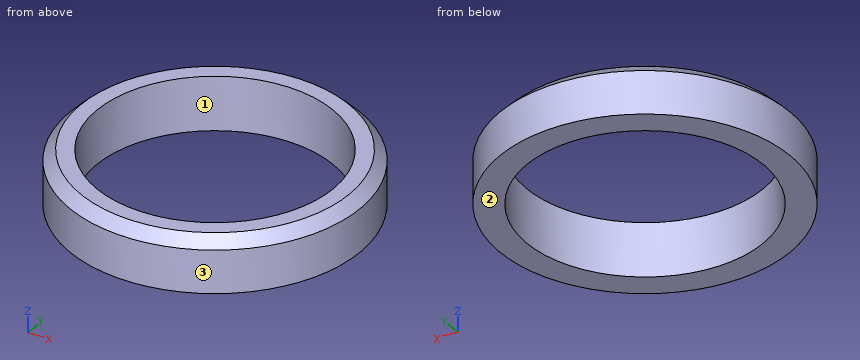
```python
from build123d import *

# Parameters (mm, degrees)
SKETCH_1_R          = 67.5
EXTRUDE_1_DEPTH     = 25
CHAMFER_1_SIZE      = 5
SKETCH_2_R          = 55
CUT_EXTRUDE_1_DEPTH = 99.67877178


with BuildPart() as part:
    # Эскиз1 → Бобышка-Вытянуть1 (new body)
    with BuildSketch(Plane.XY):
        Circle(SKETCH_1_R)
    extrude(amount=EXTRUDE_1_DEPTH)

    # Фаска1
    chamfer_1_edges = [part.edges().sort_by_distance(p)[0] for p in [
        (-67.5, 0, 25),
    ]]
    chamfer(chamfer_1_edges, length=CHAMFER_1_SIZE)

    # Эскиз2 → Вырез-Вытянуть1 (cut, through all)
    with BuildSketch(Plane(origin=(0, 0, 0), x_dir=(-1, 0, 0), z_dir=(0, 0, -1))):
        Circle(SKETCH_2_R)
    extrude(amount=-CUT_EXTRUDE_1_DEPTH, mode=Mode.SUBTRACT)


solid = part.part
```
Can you work these out from the model? Positions are in its coordinate system, mm. Face numbers are marked on the shaded views. Give positions to 0.01 mm unless a question says otherwise; leave off trailing zeros. Write each loop counter-clockwise with the first axis right and the second up, starting at its lowest first coordinate (ties: lowest second). Pieces come first, ordered by that corner, then holes. Notation, with made-up numbers: (75.25, 49.5) -> (121.25, 49.5) arc R20 cw to (121.25, 69.5) -> close; hole circle Ø5 at (27.5, 30.5). An arc over 180 degrees is marked (long way). Write item = value, one per line.
(1) I'm going to push flat-ended pins straight in: P1, Ø4, axis at x = 46.5, y = 47.5, coming from the -Z side; P2, Ø10, axis at x = -51, z = 9, coming from the -Y side; P3, Ø1.5, axis at y = -4, z = 16.5, coming from the -X side; P4, Ø10, axis at y = -6, z = 6.5, coming from the +X side. Where does each tip first touch, or does it pass through?
Worked out:
P1 = 0
P2 = -49.4
P3 = -67.42
P4 = 67.49
(2) Suppose I cut it at A-A on x = 0. Write out the boundary of the cut face in (y, z).
Worked out:
outline = (-67.5, 0) -> (-55, 0) -> (-55, 25) -> (-62.5, 25) -> (-67.5, 20) -> close; (55, 0) -> (67.5, 0) -> (67.5, 20) -> (62.5, 25) -> (55, 25) -> close
(3) Thinking about a two-plate mould opening in X: for the marked faces 1, 2 and 3, which applies, released by +X, released by -X, zero draft, split by the parting line, or undercut?
Worked out:
face_1 = undercut
face_2 = zero draft
face_3 = split by the parting line
(4) Suppose I cut it at C-C on z = 16. Write out the boundary of the cut face in (x, y).
Worked out:
outline = circle Ø135 at (0, 0); hole circle Ø110 at (0, 0)
(5) I need wall thicknesses on probe 1 along Y at (x, z) = (0, 5.5); probe 2 along X at (y, z) = (-6.5, 11.25); probe 3 along X at (y, z) = (-51, 10). Which ranges of each line are inside material? Lowest first, please. Write a range as from..to.
Worked out:
probe_1 = -67.5..-55, 55..67.5
probe_2 = -67.19..-54.61, 54.61..67.19
probe_3 = -44.22..-20.59, 20.59..44.22
